Design review of the part shown in the three views and the two pictorial views. Dimensions are in mm from the part's minimum x, y and z. A direction names the side the tool comes from. Round coordinates to 2 decimals unless told otherwise and drop trailing zeros. Loops run counter-clockwise (first coordinate to the right, second up) from the corner with the lowest first, then second, coordinate; pieces in that order, holes last.
1) Take a section at D-D (x = 9.25). State the section outline as (y, z) points, then the cut area to 3 significant figures.
2) Mouldability with a two-part tool opening along X and no side actions: class the marked faces 3, 4, 5 and 6 as pulls with the +X half, pulls with the -X half, needs draft (parallel to the pull), parting line crosses it, or undercut.
3) Take a section at A-A (y = 7.75). State the section outline as (x, z) points, then the cut area to 3 significant figures.
4) Take a section at B-B (x = 2.25). State the section outline as (y, z) points.
5) Take a section at C-C (z = 0.9). State the section outline as (x, y) points, then the cut area to 3 significant figures.
6) Insertion check: pin 1 (0.9 mm diameter, centred on x = 9, z = 1, fed in from +Y). The pin has a flat end and moves straight along its axis. Give the tip position at first contact, or say it passes through.
7) Wall thickness on L1, parallel to Y at x = 2.75, z = 1.55; L2, parallel to X at y = 8.25, z = 0.25; L3, parallel to X at y = 7.75, z = 2.35: over which ranges is each line inside the solid? List them lowest first.
8) Tool access review of the marked faces 1 and 2: name each direction out of +Z, -Z, +X, -X, +Y, -Y from which nothing blocks a thin tool from reaching the whole face with its end or side.
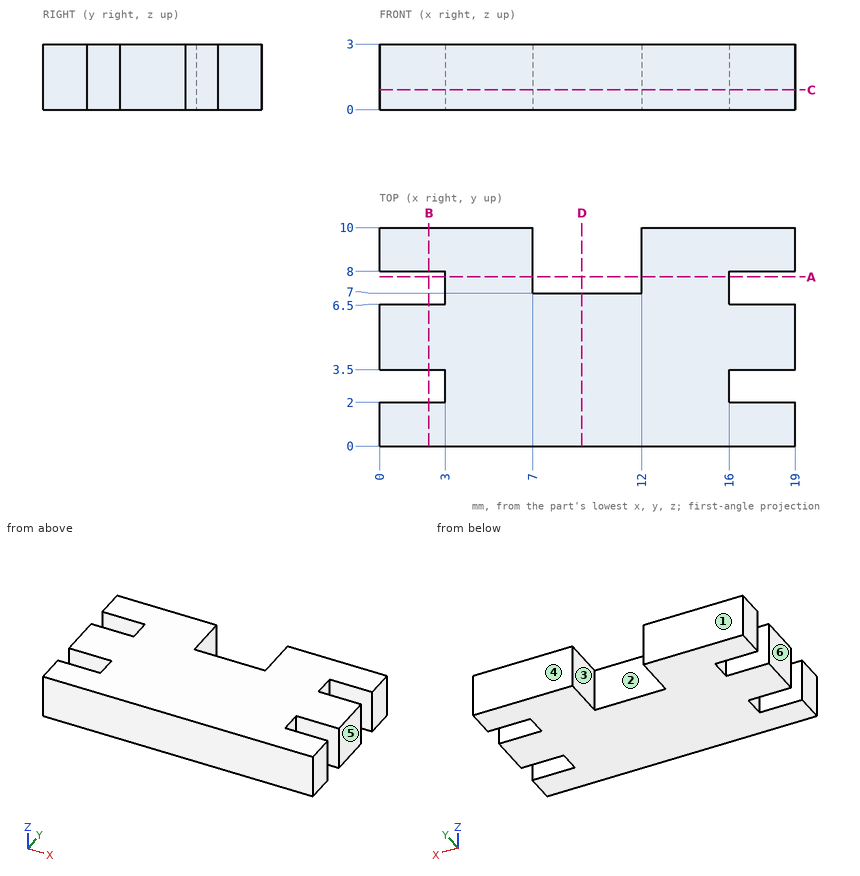
Response:
1. outline: (0, 0) - (7, 0) - (7, 3) - (0, 3) - close
1. area: 21.0 mm2
2. face 3: undercut
2. face 4: needs draft
2. face 5: pulls with the +X half
2. face 6: pulls with the -X half
3. outline: (3, 0) - (7, 0) - (7, 3) - (3, 3) - close; (12, 0) - (16, 0) - (16, 3) - (12, 3) - close
3. area: 24.0 mm2
4. outline: (0, 0) - (2, 0) - (2, 3) - (0, 3) - close; (3.5, 0) - (6.5, 0) - (6.5, 3) - (3.5, 3) - close; (8, 0) - (10, 0) - (10, 3) - (8, 3) - close
5. outline: (0, 0) - (19, 0) - (19, 2) - (16, 2) - (16, 3.5) - (19, 3.5) - (19, 6.5) - (16, 6.5) - (16, 8) - (19, 8) - (19, 10) - (12, 10) - (12, 7) - (7, 7) - (7, 10) - (0, 10) - (0, 8) - (3, 8) - (3, 6.5) - (0, 6.5) - (0, 3.5) - (3, 3.5) - (3, 2) - (0, 2) - close
5. area: 157 mm2
6. pin 1: stops at y = 7
7. L1: y = 0 to 2, 3.5 to 6.5, 8 to 10
7. L2: x = 0 to 7, 12 to 19
7. L3: x = 3 to 7, 12 to 16
8. face 1: +Z, -Z, +X, -X, +Y
8. face 2: +Z, -Z, +Y
